Here's the drawing with two shaded views (mm, measured from the low corner). I have some questions. A direction names the side the tool comes from. Give positions to 0.01 mm unless a question says otherwise; leave off trailing zeros. Loops run counter-clockwise (first coordinate to the right, second up) from the corner with the lowest first, then second, coordinate; pieces in that order, holes last. Notation, with made-up numbers: (82, 13.25) -> (118, 13.25) arc R30 ccw to (118, 37.25) -> close; hole circle Ø9 at (89.5, 54.25). An arc over 180 degrees is marked (long way). Write each question's results on one line, items separated by ' | '. Start each with the question number.
Q1. If we section it at C-C, the plane y = 6.5: List the corners of the cut face in (x, z) for me.
Q2. If I drill on line 1 along X through (y, z) = (18, 2.75); line 2 along Y through (x, z) = (9.75, 15), over which ranges is the centre line in solid material (lowest first)?
Q3. If we section it at B-B, the plane x = 10.5: List the corners of the cut face in (y, z) for me.
Q4. If we section it at D-D, the plane z = 14.25: List the corners of the cut face in (x, y) for me.
Q5. Will these pins go through, and if not, where does the flat tip stop? P1, Ø3, axis at x = 7, z = 7, coming from the +Y side; P2, Ø8, axis at x = 13.5, y = 12.5, coming from the +Z side; P3, Ø8, axis at y = 17.5, z = 5, coming from the -X side.
Q6. If we section it at A-A, the plane z = 6.5: List the corners of the cut face in (x, y) for me, plus the area to 3 significant figures.
Q7. Which directions (+Z, -Z, +X, -X, +Y, -Y) give clear straight access to the entire face, cutting with the end or side of a thin tool? Please do the marked faces 1, 2 and 3.
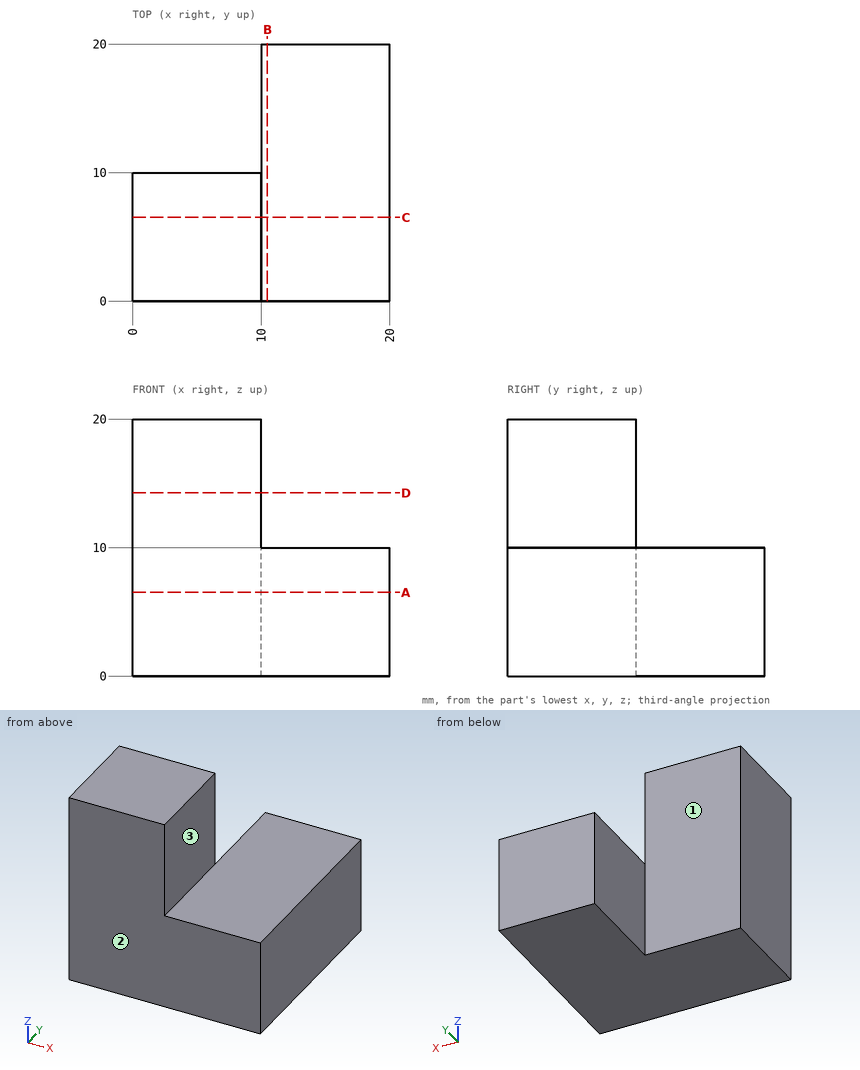
Final values:
1) outline: (0, 0) -> (20, 0) -> (20, 10) -> (10, 10) -> (10, 20) -> (0, 20) -> close
2) line 1: x = 10 to 20 | line 2: y = 0 to 10
3) outline: (0, 0) -> (20, 0) -> (20, 10) -> (0, 10) -> close
4) outline: (0, 0) -> (10, 0) -> (10, 10) -> (0, 10) -> close
5) P1: stops at y = 10 | P2: stops at z = 10 | P3: stops at x = 10
6) outline: (0, 0) -> (20, 0) -> (20, 20) -> (10, 20) -> (10, 10) -> (0, 10) -> close | area: 300 mm²
7) face 1: +Z, -Z, -X, +Y | face 2: +Z, -Z, +X, -X, -Y | face 3: +Z, +X, +Y, -Y
